Verification items for the finished model (mm, model axes). Face numbers are marked on the shaded views. A direction names the side the tool comes from. Round coordinates to 2 decimals unless told otherwise and drop trailing zeros. Write each loop counter-clockwise with the first axis right and the second up, starting at its lowest first coordinate (ties: lowest second). Pieces come first, ordered by that corner, then holes. Notation, with made-up numbers: M 7,-1 L 34,-1 A29 ccw 34,38 Z; hole C 59.5,79 d8. An arc over 180 degrees is marked long. Answer in a Markdown table with one row per item. Add a question column.
1. Material ranges on probe 1 along Y at (x, z) = (3.5, -1.25); probe 2 along X at (y, z) = (0.45, -3.75); probe 3 along Y at (x, z) = (4, -4.5), recorded low to high.
2. Sectioned sample at C-C on x = 4. Record the cut outline in (y, z), plus the area to 3 significant figures.
3. Go/stop test with flat-tipped pins: pin 1 Ø2 at (x, z) = (5.5, -4) entering from -Y; pin 2 Ø1 at (x, y) = (2, -1) entering from +Z. Record where each tip stops, or that it passes through.
4. Draft check along X on the marked faces 4, 5 and 6. Enter one of: pulls with the +X half, pulls with the -X half, needs draft (parallel to the pull), parting line crosses it, or undercut.
5. Sectioned sample at A-A on y = 0.45. Record the cut outline in (x, z).
6. Sectioned sample at D-D on y = 1.3. Record the cut outline in (x, z).
7. Set-up check for the marked faces 1, 2 and 3: record each of +Z, -Z, +X, -X, +Y, -Y from which the full face is reachable in a straight line by a thin tool's end or side.
8. Sectioned sample at B-B on z = -3.75. Record the cut outline in (x, y).
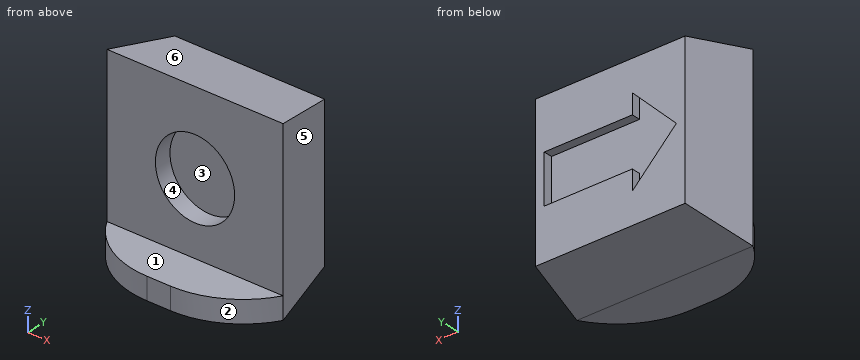
```python
from build123d import *

# Parameters (mm, degrees)
SKETCH1_W               = 8
SKETCH1_H               = 8
BOSS_EXTRUDE1_DEPTH     = 3
CUT_EXTRUDE1_DEPTH      = 12.704699911
CUT_EXTRUDE1_DEPTH_BACK = 12.704699911
CUT_EXTRUDE2_DEPTH      = 11
SKETCH4_R               = 1.8
CUT_EXTRUDE3_DEPTH      = 0.8
SKETCH5_W               = 8
SKETCH5_H               = 1
BOSS_EXTRUDE2_DEPTH     = 2
FILLET1_R               = 4
SKETCH6_W               = 4
SKETCH6_H               = 2.2
CUT_EXTRUDE4_DEPTH      = 0.4


with BuildPart() as part:
    # Sketch1 → Boss-Extrude1 (new body)
    with BuildSketch(Plane(origin=(0, 0, 0), x_dir=(1, 0, 0), z_dir=(0, 1, 0))):
        with Locations((4, 4)):
            Rectangle(SKETCH1_W, SKETCH1_H)
    extrude(amount=BOSS_EXTRUDE1_DEPTH)

    # Sketch2 → Cut-Extrude1 (cut, two sides: drawn at the far end of the back side and taken through both)
    with BuildSketch(Plane.XY.offset(-CUT_EXTRUDE1_DEPTH_BACK)):
        Polygon((0, 0), (0.6, 3), (0, 3), align=None)
        Polygon((8, 0), (7.4, 3), (8, 3), align=None)
    extrude(amount=CUT_EXTRUDE1_DEPTH + CUT_EXTRUDE1_DEPTH_BACK, mode=Mode.SUBTRACT)

    # Sketch3 → Cut-Extrude2 (cut)
    with BuildSketch(Plane(origin=(0, 0, 0), x_dir=(0, 0, -1), z_dir=(1, 0, 0))):
        Polygon((0, 0), (0.6, 3), (0, 3), align=None)
        Polygon((8, 3), (7.4, 3), (8, 0), align=None)
    extrude(amount=CUT_EXTRUDE2_DEPTH, mode=Mode.SUBTRACT)

    # Sketch4 → Cut-Extrude3 (cut)
    with BuildSketch(Plane.XZ):
        with Locations(Location((4, -3.75, 0), (0, 0, 270))):
            Circle(SKETCH4_R)
    extrude(amount=-CUT_EXTRUDE3_DEPTH, mode=Mode.SUBTRACT)

    # Sketch5 → Boss-Extrude2 (add)
    with BuildSketch(Plane.XZ):
        with Locations((4, -7.5)):
            Rectangle(SKETCH5_W, SKETCH5_H)
    extrude(amount=BOSS_EXTRUDE2_DEPTH)

    # Fillet1
    # the kernel refuses this fillet: 4 mm, written as the material it takes off along each edge
    with BuildSketch(Plane(origin=(8, -2, -16.660254038), x_dir=(0, 1, 0), z_dir=(0, 0, 1)), Plane(origin=(0, -2, 1.660254038), x_dir=(0, 1, 0), z_dir=(0, 0, -1))) as fillet1_piece_1:
        with BuildLine():
            CenterArc((4, 3.464101615), FILLET1_R, 180, 60)
            Line((0, 3.464101615), (-0.08, 3.464101615))
            Line((-0.08, 3.464101615), (-0.08, 0))
            Line((-0.08, 0), (0, -0.08))
            ThreePointArc((0, -0.08), (1, -0.08), (1.96, -0.069282032))
            Line((1.96, -0.069282032), (2, 0))
        make_face()
    extrude(amount=18.320508076, mode=Mode.SUBTRACT)

    # Sketch6 → Cut-Extrude4 (cut)
    with BuildSketch(Plane(origin=(0, 3, 0), x_dir=(1, 0, 0), z_dir=(0, 1, 0))):
        Polygon((1, 4), (3, 2), (3, 2.9), (3, 5.1), (3, 6), align=None)
        with Locations((5, 4)):
            Rectangle(SKETCH6_W, SKETCH6_H)
    extrude(amount=-CUT_EXTRUDE4_DEPTH, mode=Mode.SUBTRACT)


solid = part.part
```
Geometry check:
| question | item | result |
|---|---|---|
| 1 | probe 1 | y = 0 to 3 |
| 1 | probe 2 | x = 0.09 to 2.2, 5.8 to 7.91 |
| 1 | probe 3 | y = 0.8 to 2.6 |
| 2 | outline | M -2,-8 L 0,-8 L 3,-7.4 L 3,-5.1 L 2.6,-5.1 L 2.6,-2.9 L 3,-2.9 L 3,-0.6 L 0,0 L 0,-1.95 L 0.8,-1.95 L 0.8,-5.55 L 0,-5.55 L 0,-7 L -2,-7 Z |
| 2 | area | 20.4 mm2 |
| 3 | pin 1 | stops at y = 0 |
| 3 | pin 2 | stops at z = -7 |
| 4 | face 4 | undercut |
| 4 | face 5 | pulls with the +X half |
| 4 | face 6 | needs draft |
| 5 | outline | M 0.09,-7.91 L 7.91,-7.91 L 7.91,-0.09 L 0.09,-0.09 Z; hole C 4,-3.75 d3.6 |
| 6 | outline | M 0.26,-7.74 L 7.74,-7.74 L 7.74,-0.26 L 0.26,-0.26 Z |
| 7 | face 1 | +Z, +X, -X, -Y |
| 7 | face 2 | +Z, -Z, +X, -Y |
| 7 | face 3 | -Y |
| 8 | outline | M 0,0 L 2.2,0 L 2.2,0.8 L 5.8,0.8 L 5.8,0 L 8,0 L 7.4,3 L 7,3 L 7,2.6 L 1.25,2.6 L 1.25,3 L 0.6,3 Z |
